CAD build for the part. Positions are in the model's coordinates, mm. A direction names the side the tool comes from. Coordinates: 2 decimals unless noted, no trailing zeros. Loops run counter-clockwise (first coordinate to the right, second up) from the corner with the lowest first, then second, coordinate; pieces in that order, holes last. Notation, with made-up numbers: (8.5, 64) -> (67.5, 64) arc R16 cw to (67.5, 72) -> close; hole circle Ø2 at (56.5, -6). An arc over 180 degrees is marked (long way). Answer as a JSON object with one key per item and string values. Group by question number.
from build123d import *

# Parameters (mm, degrees)
BOSS_EXTRUDE1_DEPTH = 7.62
CUT_EXTRUDE1_REACH  = 9.62
SKETCH3_R           = 1.7526


with BuildPart() as part:
    # Sketch1 → Boss-Extrude1 (new body)
    with BuildSketch(Plane(origin=(0, 0, 0), x_dir=(1, 0, 0), z_dir=(0, 1, 0))):
        with BuildLine():
            Line((-117.31625, 0), (-117.31625, -7.62))
            Line((-117.31625, -7.62), (-77.43825, -7.62))
            Line((-77.43825, -7.62), (-77.43825, 0))
            ThreePointArc((-77.43825, 0), (0, 77.43825), (77.43825, 0))
            Line((77.43825, 0), (77.43825, -7.62))
            Line((77.43825, -7.62), (117.31625, -7.62))
            Line((117.31625, -7.62), (117.31625, 0))
            ThreePointArc((117.31625, 0), (0, 117.31625), (-117.31625, 0))
        make_face()
    extrude(amount=BOSS_EXTRUDE1_DEPTH)

    # Sketch3 → Cut-Extrude1 (cut, up to next)
    with BuildSketch(Plane(origin=(0, 7.62, 0), x_dir=(1, 0, 0), z_dir=(0, 1, 0)), mode=Mode.PRIVATE) as cut_extrude1_sk1:
        with Locations((-109.69625, -3.81)):
            Circle(SKETCH3_R)
    cut_extrude1_tool1 = extrude(cut_extrude1_sk1.sketch, amount=-CUT_EXTRUDE1_REACH, mode=Mode.PRIVATE) & part.part
    add(cut_extrude1_tool1.solids().sort_by_distance((-109.69625, 7.62, 3.81))[0], mode=Mode.SUBTRACT)
    # Sketch3 → Cut-Extrude1 (cut, up to next)
    with BuildSketch(Plane(origin=(0, 7.62, 0), x_dir=(1, 0, 0), z_dir=(0, 1, 0)), mode=Mode.PRIVATE) as cut_extrude1_sk2:
        with Locations((-85.05825, -3.81)):
            Circle(SKETCH3_R)
    cut_extrude1_tool2 = extrude(cut_extrude1_sk2.sketch, amount=-CUT_EXTRUDE1_REACH, mode=Mode.PRIVATE) & part.part
    add(cut_extrude1_tool2.solids().sort_by_distance((-85.05825, 7.62, 3.81))[0], mode=Mode.SUBTRACT)
    # Sketch3 → Cut-Extrude1 (cut, up to next)
    with BuildSketch(Plane(origin=(0, 7.62, 0), x_dir=(1, 0, 0), z_dir=(0, 1, 0)), mode=Mode.PRIVATE) as cut_extrude1_sk3:
        with Locations((85.05825, -3.81)):
            Circle(SKETCH3_R)
    cut_extrude1_tool3 = extrude(cut_extrude1_sk3.sketch, amount=-CUT_EXTRUDE1_REACH, mode=Mode.PRIVATE) & part.part
    add(cut_extrude1_tool3.solids().sort_by_distance((85.05825, 7.62, 3.81))[0], mode=Mode.SUBTRACT)
    # Sketch3 → Cut-Extrude1 (cut, up to next)
    with BuildSketch(Plane(origin=(0, 7.62, 0), x_dir=(1, 0, 0), z_dir=(0, 1, 0)), mode=Mode.PRIVATE) as cut_extrude1_sk4:
        with Locations((109.69625, -3.81)):
            Circle(SKETCH3_R)
    cut_extrude1_tool4 = extrude(cut_extrude1_sk4.sketch, amount=-CUT_EXTRUDE1_REACH, mode=Mode.PRIVATE) & part.part
    add(cut_extrude1_tool4.solids().sort_by_distance((109.69625, 7.62, 3.81))[0], mode=Mode.SUBTRACT)
    # Sketch3 → Cut-Extrude1 (cut, up to next)
    with BuildSketch(Plane(origin=(0, 7.62, 0), x_dir=(1, 0, 0), z_dir=(0, 1, 0)), mode=Mode.PRIVATE) as cut_extrude1_sk5:
        with Locations((31.75, 82.55)):
            Circle(SKETCH3_R)
    cut_extrude1_tool5 = extrude(cut_extrude1_sk5.sketch, amount=-CUT_EXTRUDE1_REACH, mode=Mode.PRIVATE) & part.part
    add(cut_extrude1_tool5.solids().sort_by_distance((31.75, 7.62, -82.55))[0], mode=Mode.SUBTRACT)
    # Sketch3 → Cut-Extrude1 (cut, up to next)
    with BuildSketch(Plane(origin=(0, 7.62, 0), x_dir=(1, 0, 0), z_dir=(0, 1, 0)), mode=Mode.PRIVATE) as cut_extrude1_sk6:
        with Locations((63.5, 82.55)):
            Circle(SKETCH3_R)
    cut_extrude1_tool6 = extrude(cut_extrude1_sk6.sketch, amount=-CUT_EXTRUDE1_REACH, mode=Mode.PRIVATE) & part.part
    add(cut_extrude1_tool6.solids().sort_by_distance((63.5, 7.62, -82.55))[0], mode=Mode.SUBTRACT)
    # Sketch3 → Cut-Extrude1 (cut, up to next)
    with BuildSketch(Plane(origin=(0, 7.62, 0), x_dir=(1, 0, 0), z_dir=(0, 1, 0)), mode=Mode.PRIVATE) as cut_extrude1_sk7:
        with Locations((63.5, 55.812428263)):
            Circle(SKETCH3_R)
    cut_extrude1_tool7 = extrude(cut_extrude1_sk7.sketch, amount=-CUT_EXTRUDE1_REACH, mode=Mode.PRIVATE) & part.part
    add(cut_extrude1_tool7.solids().sort_by_distance((63.5, 7.62, -55.812428))[0], mode=Mode.SUBTRACT)
    # Sketch3 → Cut-Extrude1 (cut, up to next)
    with BuildSketch(Plane(origin=(0, 7.62, 0), x_dir=(1, 0, 0), z_dir=(0, 1, 0)), mode=Mode.PRIVATE) as cut_extrude1_sk8:
        with Locations((95.25, 55.812428263)):
            Circle(SKETCH3_R)
    cut_extrude1_tool8 = extrude(cut_extrude1_sk8.sketch, amount=-CUT_EXTRUDE1_REACH, mode=Mode.PRIVATE) & part.part
    add(cut_extrude1_tool8.solids().sort_by_distance((95.25, 7.62, -55.812428))[0], mode=Mode.SUBTRACT)


solid = part.part
Item 1: Band-saw the part on B-B, the plane y = 6. Count the separate pieces of the cut face and the enclosed holes in it, and give its area (3 significant figures).
Item 2: 3-axis set-ups, long thin cutter, end or side, ignore diameter. For faces 5 (the flat face through (77.438, 4, 4)), 6 (the flat face through (-2, 0, -83)): which of +Z, -Z, +X, -X, +Y, -Y reach the whole face in a straight line?
Item 3: Band-saw the part on D-D, the plane z = -90. List the corners of the cut face in (x, y), and give its area (3 significant figures).
Item 4: Pull direction X, two halves, no side cores. Call faces 1 (the flat face through (-98, 4, 7.62)), 2 (the cylindrical face through (2.58, 3.757, -117.288)), 3 (the flat face through (-77.438, 4, 4)), 4 (the flat face through (-117.316, 4, 4)): +X half, -X half, draft (parallel to the pull), parting line (faces both ways), or undercut.
Item 5: Drill centre lines: L1, parallel to X at y = 2, z = 3.81; L2, parallel to X at y = 5.75, z = -84; L3, parallel to Z at x = 63.5, y = 5. Where is each one in solid material? Low to high.
Item 6: Band-saw the part on A-A, the plane z = -47.5. List the corners of the cut face in (x, y), and give its area (3 significant figures).
Item 7: Band-saw the part on C-C, the plane x = -103. List the corners of the cut face in (y, z), and give its area (3 significant figures).
Item 8: Flat gauge pins, fed straight in: P1, Ø3, axis at x = 63.5, z = -55.81, coming from the +Y side; P2, Ø4.5, axis at x = 95.25, z = -55.81, coming from the -Y side; P3, Ø4, axis at y = 4.5, z = -91, coming from the +X side; P4, Ø1.5, axis at y = 1, z = -45, coming from the +X side. Where does each tip first touch, or does it go through?
Reply:
{
 "1": {"separate pieces": "1", "enclosed holes": "8", "area": "12,700 mm²"},
 "2": {"face 5": "+Z, +Y, -Y", "face 6": "+Z, -Z, +X, -X, -Y"},
 "3": {"outline": "(-75.25, 0) -> (75.25, 0) -> (75.25, 7.62) -> (-75.25, 7.62) -> close", "area": "1,150 mm²"},
 "4": {"face 1": "draft", "face 2": "parting line", "face 3": "undercut", "face 4": "-X half"},
 "5": {"L1": "-117.32 to -111.45, -107.94 to -86.81, -83.31 to -77.44, 77.44 to 83.31, 86.81 to 107.94, 111.45 to 117.32", "L2": "-81.9 to 30.77, 32.73 to 62.52, 64.48 to 81.9", "L3": "-98.65 to -84.3, -80.8 to -57.57, -54.06 to -44.32"},
 "6": {"outline": "(-107.27, 0) -> (-61.16, 0) -> (-61.16, 7.62) -> (-107.27, 7.62) -> close; (61.16, 0) -> (107.27, 0) -> (107.27, 7.62) -> (61.16, 7.62) -> close", "area": "703 mm²"},
 "7": {"outline": "(0, -56.16) -> (7.62, -56.16) -> (7.62, 7.62) -> (0, 7.62) -> close", "area": "486 mm²"},
 "8": {"P1": "through", "P2": "y = 0", "P3": "x = 76.43", "P4": "x = 108.65"}
}
